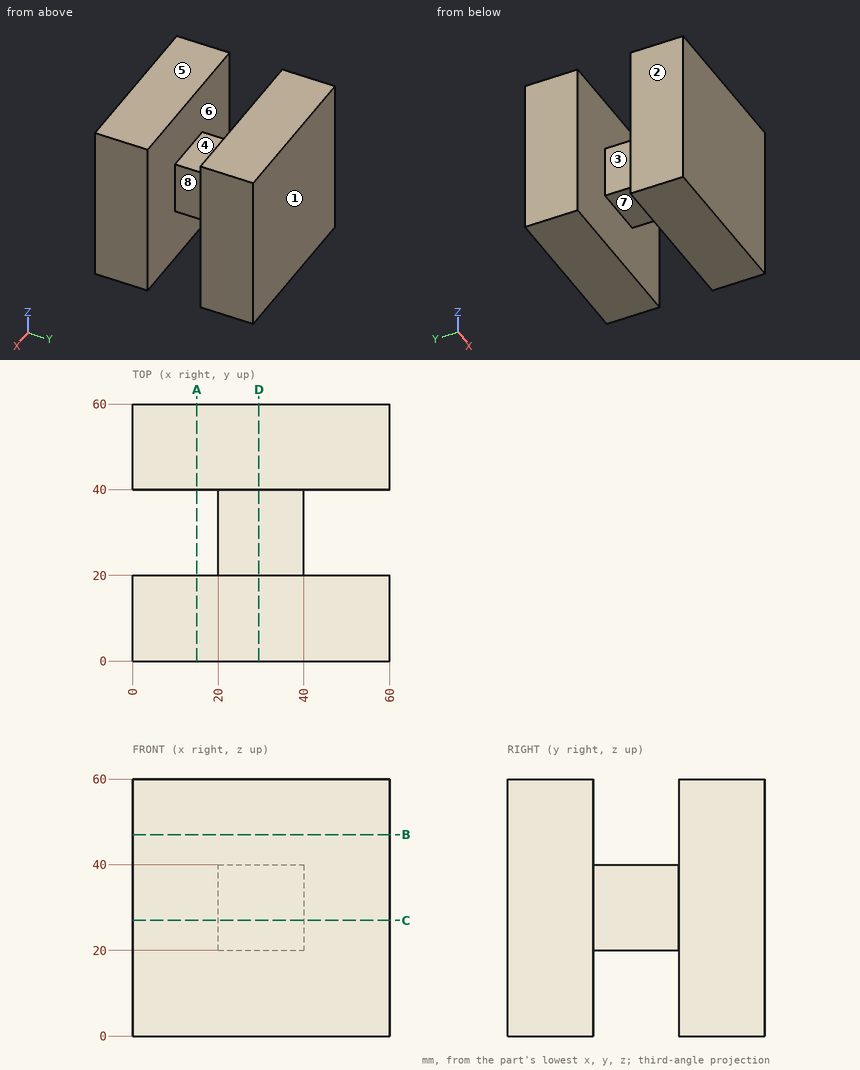
The drawing under review shows one solid part. Ordinate dimensions are in mm from its lowest x, y, z. A direction names the side the tool comes from. Give positions to 0.01 mm unless a question says otherwise; leave off trailing zeros. Order: outer loops, then holes, each group sorted by start corner. A loop starts at its lowest first (then second) coordinate and runs counter-clockwise, first axis right, second up. Notation, with made-up numbers: (13.25, 70.5) -> (57.25, 70.5) arc R22 cw to (57.25, 100.5) -> close; hole circle Ø7 at (50, 31.25). An arc over 180 degrees is marked (long way). Write item = value, one per line.
1) Draft analysis for pull direction Y (two halves, no side actions). For the marked faces 1, 2 and 3, state which applies: pulls with the +Y half, pulls with the -Y half, needs draft (parallel to the pull), parting line crosses it, or undercut.
Findings:
face_1 = pulls with the +Y half
face_2 = needs draft
face_3 = undercut
2) We need section A-A, the plane x = 15. Give the boundary of the cut face in (y, z).
Findings:
outline = (0, 0) -> (20, 0) -> (20, 60) -> (0, 60) -> close; (40, 0) -> (60, 0) -> (60, 60) -> (40, 60) -> close
3) We need section B-B, the plane z = 47. Give the boundary of the cut face in (x, y).
Findings:
outline = (0, 0) -> (60, 0) -> (60, 20) -> (0, 20) -> close; (0, 40) -> (60, 40) -> (60, 60) -> (0, 60) -> close
4) We need section C-C, the plane z = 27. Give the boundary of the cut face in (x, y), and give its area (3 significant figures).
Findings:
outline = (0, 0) -> (60, 0) -> (60, 20) -> (40, 20) -> (40, 40) -> (60, 40) -> (60, 60) -> (0, 60) -> (0, 40) -> (20, 40) -> (20, 20) -> (0, 20) -> close
area = 2,800 mm^2
5) Insertion check: pin 1 (10 mm diameter, centred on x = 29.5, y = 34, fed in from -Z); pin 2 (6 mm diameter, centred on y = 33, z = 27.5, fed in from -X); pin 3 (6 mm diameter, centred on y = 31.5, z = 28, fed in from +X). Each pin has a flat end and moves straight along its axis. Give the tip position at first contact, or say it passes through.
Findings:
pin_1 = 20
pin_2 = 20
pin_3 = 40
6) To check wall thickness, follow L1, parallel to Y at x = 54, z = 18.5; L2, parallel to X at y = 22.5, z = 38.5. State the ranges of each line that lie inside material, in increasing order. Write a range as from..to.
Findings:
L1 = 0..20, 40..60
L2 = 20..40
7) For the marked faces 4, 5, 6, 7 and 8, list the 3-axis set-ups (+Z, -Z, +X, -X, +Y, -Y) from which the entire face can be reached by the end or side of a thin tool; tool diameter is ignored.
Findings:
face_4 = +Z, +X, -X
face_5 = +Z, +X, -X, +Y, -Y
face_6 = none
face_7 = -Z, +X, -X
face_8 = +Z, -Z, +X
8) We need section D-D, the plane x = 29.5. Give the boundary of the cut face in (y, z), and give its area (3 significant figures).
Findings:
outline = (0, 0) -> (20, 0) -> (20, 20) -> (40, 20) -> (40, 0) -> (60, 0) -> (60, 60) -> (40, 60) -> (40, 40) -> (20, 40) -> (20, 60) -> (0, 60) -> close
area = 2,800 mm^2
